Verification items for this drawing (mm, ordinates from the low corner). A direction names the side the tool comes from. Round coordinates to 2 decimals unless told otherwise and drop trailing zeros. Order: outer loops, then holes, each group sorted by start corner. A loop starts at its lowest first (then second) coordinate and runs counter-clockwise, first axis right, second up.
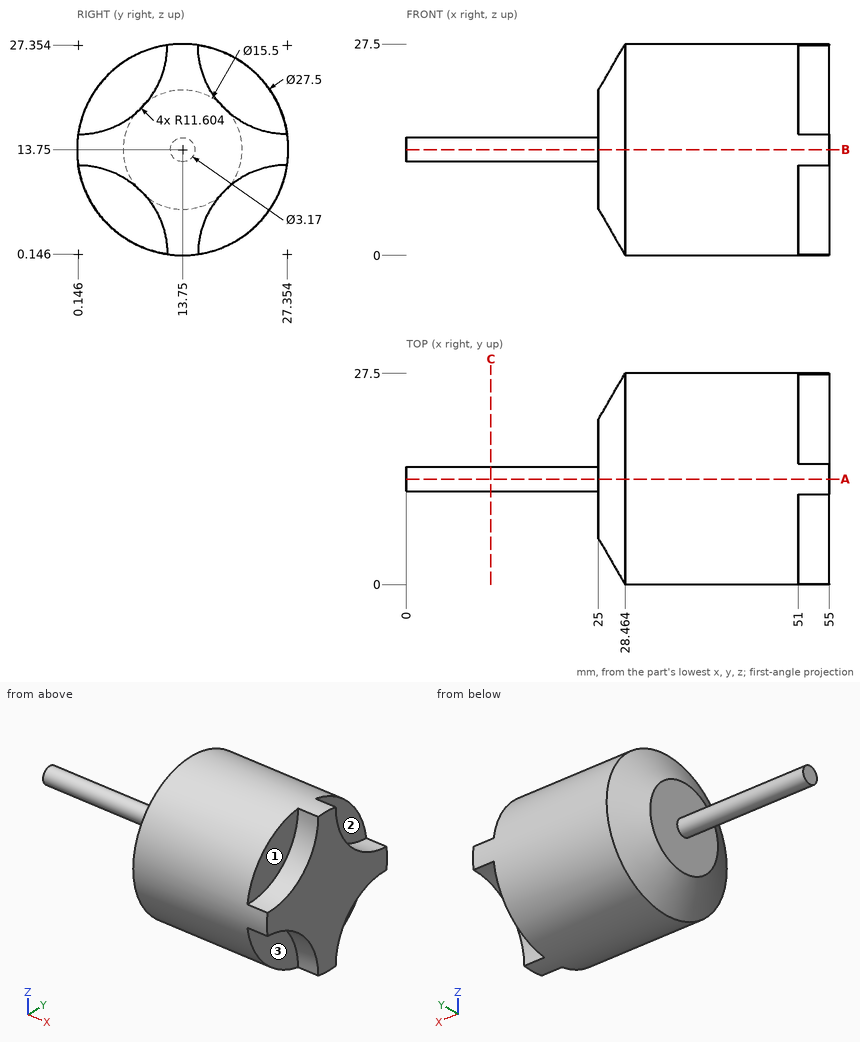
Item 1: Go/stop test with flat-tipped pins: P1, Ø3.5, axis at y = 19, z = 22.5, coming from the +X side; P2, Ø10, axis at y = 21, z = 23.5, coming from the -X side; P3, Ø2, axis at x = 37, z = 4.5, coming from the -Y side. Record where each tip stops, or that it passes through.
Answer:
P1: stops at x = 51
P2: stops at x = 25
P3: stops at y = 2.75
Item 2: Access from +Z, -Z, +X, -X, +Y, -Y to the whole of each face (thin tool, end or side, straight path). Record for the marked faces 1, 2 and 3.
Answer:
face 1: +Z, +X, -Y
face 2: +Z, +X, +Y
face 3: -Z, +X, -Y
Item 3: Sectioned sample at A-A (y = 13.75). Record the cut outline in (x, z) (1 decimal).
Answer:
outline: (0, 12.2) - (25, 12.2) - (25, 6) - (28.5, 0) - (55, 0) - (55, 27.5) - (28.5, 27.5) - (25, 21.5) - (25, 15.3) - (0, 15.3) - close
Item 4: Scan lines: line 1 along Y through (x, z) = (48, 13.25); line 2 along X through (y, z) = (11, 7.75); line 3 along X through (y, z) = (15.5, 4.75). Record each from-to range of solid material in increasing order.
Answer:
line 1: y = 0.01 to 27.49
line 2: x = 25 to 55
line 3: x = 25.82 to 55
Item 5: Sectioned sample at C-C (x = 11). Record the cut outline in (y, z) (3 decimals).
Answer:
outline: circle Ø3.17 at (13.75, 13.75)
